Read the model definition and answer for the solid it produces. Units are mm, in the model's axes. Coordinates: 2 decimals unless noted, no trailing zeros. Order: outer loops, then holes, each group sorted by start corner. A loop starts at its lowest first (then second) coordinate and runs counter-clockwise, first axis right, second up. Notation, with made-up numbers: M 58.5,33 L 83.5,33 A26 cw 83.5,62 Z; hole C 59,22 d3. An arc over 180 degrees is marked long. Put each result on its own line as item: value.
from build123d import *

# Parameters (mm, degrees)
SKETCH1_R           = 38
SKETCH1_R_2         = 2.2
SKETCH1_R_3         = 28.85
SKETCH1_R_4         = 3.3
BOSS_EXTRUDE1_DEPTH = 12.7
MOVE_FACE4_BY       = 0.7


with BuildPart() as part:
    # Sketch1 → Boss-Extrude1 (new body)
    # profile 1 of 2: a face of its own
    with BuildSketch(Plane(origin=(0, 0, 0), x_dir=(0, 0, -1), z_dir=(1, 0, 0))):
        Circle(SKETCH1_R)
        with Locations((23.5, -23.5)):
            Circle(SKETCH1_R_2, mode=Mode.SUBTRACT)
        with Locations((-23.5, -23.5)):
            Circle(SKETCH1_R_2, mode=Mode.SUBTRACT)
        with Locations((23.5, 23.5)):
            Circle(SKETCH1_R_2, mode=Mode.SUBTRACT)
        with Locations((-23.5, 23.5)):
            Circle(SKETCH1_R_2, mode=Mode.SUBTRACT)
        Circle(SKETCH1_R_3, mode=Mode.SUBTRACT)
    # profile 2 of 2: a face of its own
    with BuildSketch(Plane(origin=(0, 0, 0), x_dir=(0, 0, -1), z_dir=(1, 0, 0))):
        with BuildLine():
            ThreePointArc((38, 0), (4.959995304, -37.674904732), (-36.705181399, -9.835123714))
            Line((-36.705181399, -9.835123714), (-13.791539357, -95.35))
            Line((-13.791539357, -95.35), (68.588460643, -95.35))
            Line((68.588460643, -95.35), (68.588460643, -82.65))
            Line((68.588460643, -82.65), (35.936663125, 12.351366055))
            ThreePointArc((35.936663125, 12.351366055), (37.480616315, 6.261261903), (38, 0))
        make_face()
        with Locations((15.59, -89)):
            Circle(SKETCH1_R_4, mode=Mode.SUBTRACT)
        with Locations((38.59, -89)):
            Circle(SKETCH1_R_4, mode=Mode.SUBTRACT)
        with Locations((61.59, -89)):
            Circle(SKETCH1_R_4, mode=Mode.SUBTRACT)
    extrude(amount=BOSS_EXTRUDE1_DEPTH)

    # Move Face4: a face moved inward by 0.7
    extrude(part.faces().sort_by_distance((12.7, -45.322375042, -15.580878329))[0], amount=MOVE_FACE4_BY, dir=(-1, 0, 0), mode=Mode.SUBTRACT)


solid = part.part
Q1. For a pull along Z with two mould halves and no side action, classify faces 1 (the face through (5.92, 36.57, 10.32)), 2 (the face through (12, -43, -15)), 3 (the face through (5.916, 21.352, 23.977)) as +Z half, -Z half, draft (parallel to the pull), parting line (faces both ways), or undercut.
Answers below:
face 1: parting line
face 2: draft
face 3: undercut
Q2. Find section C-C on y = -2. Write down the section's boundary in (x, z), plus the area to 3 significant figures.
Answers below:
outline: M 0,-40.87 L 12,-40.87 L 12,-28.78 L 0,-28.78 Z; M 0,28.78 L 12,28.78 L 12,37.95 L 0,37.95 Z
area: 255 mm^2
Q3. Find section A-A on x = 6. Give the number of separate pieces and of enclosed holes in the cut face, plus the area to 3 significant figures.
Answers below:
separate pieces: 1
enclosed holes: 8
area: 7,390 mm^2
Q4. Find section B-B on z = -15.59. Write down the section's boundary in (x, y), plus the area to 3 significant figures.
Answers below:
outline: M 0,-95.35 L 12,-95.35 L 12,-92.3 L 0,-92.3 Z; M 0,-85.7 L 12,-85.7 L 12,-24.27 L 0,-24.27 Z; M 0,24.27 L 12,24.27 L 12,34.65 L 0,34.65 Z
area: 898 mm^2
Q5. Given pin 1 (5 mm diameter, centred on x = 8, y = -50, fed in from +Z); pin 2 (6 mm diameter, centred on x = 7.5, z = 6, fed in from +Y); pin 3 (1.5 mm diameter, centred on x = 9.5, y = 5.5, fed in from -Z), each flat-ended and moving along its own axis, determine where each tip first touches the part or whether it passes through.
Answers below:
pin 1: stops at z = 26.61
pin 2: stops at y = 37.88
pin 3: stops at z = -38.55
Q6. Consider line 1 along Z through (x, y) = (3.25, 22.5); line 2 along Y through (x, z) = (3.5, -15.59); line 3 along Y through (x, z) = (2.5, -17). Determine where each line is inside the solid, lowest interval first.
Answers below:
line 1: z = -30.62 to -25.46, -21.54 to -18.06, 18.06 to 21.54, 25.46 to 30.62
line 2: y = -95.35 to -92.3, -85.7 to -24.27, 24.27 to 34.65
line 3: y = -95.35 to -91.98, -86.02 to -23.31, 23.31 to 33.99
Q7. Find section D-D on z = -61.59. Write down the section's boundary in (x, y).
Answers below:
outline: M 0,-95.35 L 12,-95.35 L 12,-92.3 L 0,-92.3 Z; M 0,-85.7 L 12,-85.7 L 12,-62.29 L 0,-62.29 Z
